Study the drawing (mm; zero at the part's minimum x, y, z) and answer. A direction names the side the tool comes from. Round coordinates to 2 decimals unless told otherwise and drop trailing zeros. Write each loop counter-clockwise with the first axis right and the second up, starting at its lowest first coordinate (ties: lowest second). Pieces come first, ordered by that corner, then holes.
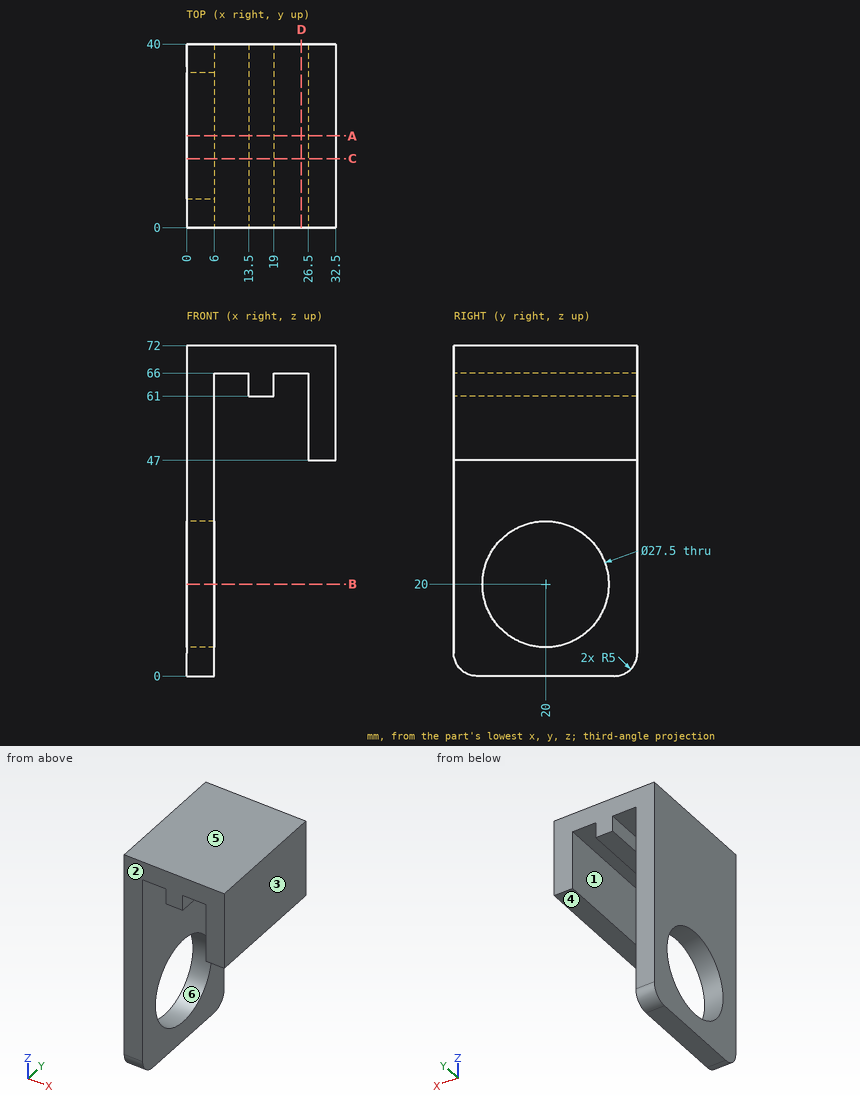
1. A tool of negligible diameter and unlimited length cuts with its end or side. For the marked faces 1 and 2, from which of +Z, -Z, +X, -X, +Y, -Y can it reach the whole face along a straight path? Write none if from no direction.
Geometry says:
face 1: -Z, +Y, -Y
face 2: +Z, -Z, +X, -X, -Y
2. Given pin 1 (5 mm diameter, centred on x = 29.5, y = 16.5, fed in from -Z); pin 2 (1.6 mm diameter, centred on x = 15, y = 29, fed in from -Z), each flat-ended and moving along its own axis, determine where each tip first touches the part or whether it passes through.
Geometry says:
pin 1: stops at z = 47
pin 2: stops at z = 61
3. Section D-D on x = 25 is taken. Determine the outline of the cut face in (y, z), plus the area to 3 significant figures.
Geometry says:
outline: (0, 66) - (40, 66) - (40, 72) - (0, 72) - close
area: 240 mm2
4. Section A-A on y = 20 is taken. Determine the outline of the cut face in (x, z), plus the area to 4 significant figures.
Geometry says:
outline: (0, 0) - (6, 0) - (6, 6.25) - (0, 6.25) - close; (0, 33.75) - (6, 33.75) - (6, 66) - (13.5, 66) - (13.5, 61) - (19, 61) - (19, 66) - (26.5, 66) - (26.5, 47) - (32.5, 47) - (32.5, 72) - (0, 72) - close
area: 567.5 mm2
5. For a pull along Z with two mould halves and no side action, classify the marked faces 3, 4, 5 and 6 as released by +Z, released by -Z, zero draft, split by the parting line, or undercut.
Geometry says:
face 3: zero draft
face 4: released by -Z
face 5: released by +Z
face 6: undercut
6. Section C-C on y = 15 is taken. Determine the outline of the cut face in (x, z).
Geometry says:
outline: (0, 0) - (6, 0) - (6, 7.19) - (0, 7.19) - close; (0, 32.81) - (6, 32.81) - (6, 66) - (13.5, 66) - (13.5, 61) - (19, 61) - (19, 66) - (26.5, 66) - (26.5, 47) - (32.5, 47) - (32.5, 72) - (0, 72) - close
7. Section B-B on z = 20 is taken. Determine the outline of the cut face in (x, y).
Geometry says:
outline: (0, 0) - (6, 0) - (6, 6.25) - (0, 6.25) - close; (0, 33.75) - (6, 33.75) - (6, 40) - (0, 40) - close
8. Straight lines are drawn through the part: line 1 along X through (y, z) = (6, 62); line 2 along Z through (x, y) = (3, 20); line 3 along X through (y, z) = (35.5, 20). For each, find the intervals that lie inside material, in ascending order.
Geometry says:
line 1: x = 0 to 6, 13.5 to 19, 26.5 to 32.5
line 2: z = 0 to 6.25, 33.75 to 72
line 3: x = 0 to 6
